Can you work these out from the model? Positions are in its coordinate system, mm. A direction names the side the tool comes from. Give positions to 0.01 mm unless a question says otherwise; leave off trailing zeros. Order: outer loops, then holes, each group sorted by start corner. A loop starts at its lowest first (then second) coordinate and runs counter-clockwise, first axis right, second up. Notation, with made-up numbers: M 66,51 L 121,51 A28 ccw 121,77 Z; hole C -11,-13 d8. An arc over 180 degrees is marked long. Use one line per item in the form item = value. Start each with the question number.
1. I want a section at B-B, the plane z = -39.5. List the corners of the cut face in (x, y) for me, and give its area (3 significant figures).
2. For faces 1 (the face through (48.57, 26.55, -25.74)), 2 (the face through (25, 29, -2)), 3 (the face through (37, 29, -30)), which set-ups out of +Z, -Z, +X, -X, +Y, -Y let a thin tool reach every point of the face, with its end or its side?
3. I want a section at A-A, the plane y = 11. List the corners of the cut face in (x, z) for me.
4. Will these pins go through, and if not, where does the flat tip stop? P1, Ø0.6, axis at x = 22.5, z = -49.5, coming from the +Y side; P2, Ø5, axis at x = 22.98, z = -29.85, coming from the -Y side; P3, Ø5, axis at x = 43.5, z = -40.5, coming from the +Y side; P4, Ø7.5, axis at x = 19.5, y = 12, coming from the -Z side.
5. We'd pull the mould along Y, two halves only. Please class faces 4 (the face through (22, 12, -50.2)), 5 (the face through (21.53, 29.51, -31.22)), 6 (the face through (25.74, 26.55, -2.43)): +Y half, -Y half, draft (parallel to the pull), parting line (faces both ways), or undercut.
6. I need wall thicknesses on L1, parallel to Z at x = 18, y = 22; L2, parallel to Z at x = 26, y = 4; L3, parallel to X at y = 16, z = -24. Which ranges of each line are inside material? Lowest first, please.
7. I want a section at C-C, the plane x = 44.25. Count the separate pieces of the cut face and the enclosed holes in it, and give its area (3 significant figures).
```python
from build123d import *

# Parameters (mm, degrees)
BOSS_EXTRUDE1_DEPTH = 30
CUT_EXTRUDE1_DEPTH  = 27
SKETCH3_R           = 1.75
SKETCH3_R_2         = 1.25
CUT_EXTRUDE2_DEPTH  = 3
SKETCH4_R           = 3
SKETCH4_R_2         = 2
CUT_EXTRUDE3_DEPTH  = 1
CUT_EXTRUDE4_DEPTH  = 2
FILLET1_R           = 5
FILLET2_R           = 1.5
SKETCH6_R           = 1
CUT_EXTRUDE5_DEPTH  = 1
CUT_EXTRUDE6_DEPTH  = 0.8


with BuildPart() as part:
    # Sketch1 → Boss-Extrude1 (new body)
    with BuildSketch(Plane(origin=(0, 0, 0), x_dir=(1, 0, 0), z_dir=(0, 1, 0))):
        with BuildLine():
            Line((8, 0), (43, 0))
            ThreePointArc((43, 0), (48.656854249, 2.343145751), (51, 8))
            Line((51, 8), (51, 43))
            ThreePointArc((51, 43), (48.656854249, 48.656854249), (43, 51))
            Line((43, 51), (8, 51))
            ThreePointArc((8, 51), (2.343145751, 48.656854249), (0, 43))
            Line((0, 43), (0, 8))
            ThreePointArc((0, 8), (2.343145751, 2.343145751), (8, 0))
        make_face()
    extrude(amount=BOSS_EXTRUDE1_DEPTH)

    # Sketch2 → Cut-Extrude1 (cut)
    with BuildSketch(Plane.XZ):
        with BuildLine():
            Line((8, -2), (43, -2))
            ThreePointArc((43, -2), (47.242640687, -3.757359313), (49, -8))
            Line((49, -8), (49, -43))
            ThreePointArc((49, -43), (47.242640687, -47.242640687), (43, -49))
            Line((43, -49), (8, -49))
            ThreePointArc((8, -49), (3.757359313, -47.242640687), (2, -43))
            Line((2, -43), (2, -8))
            ThreePointArc((2, -8), (3.757359313, -3.757359313), (8, -2))
        make_face()
    extrude(amount=-CUT_EXTRUDE1_DEPTH, mode=Mode.SUBTRACT)

    # Sketch3 → Cut-Extrude2 (cut)
    with BuildSketch(Plane.XZ.offset(-27)):
        with Locations(Location((6.75, -11.5, 0), (0, 0, 270))):
            Circle(SKETCH3_R)
        with Locations(Location((44.25, -11.5, 0), (0, 0, 90))):
            Circle(SKETCH3_R)
        with Locations(Location((44.25, -39.5, 0), (0, 0, 270))):
            Circle(SKETCH3_R)
        with Locations(Location((6.75, -39.5, 0), (0, 0, 90))):
            Circle(SKETCH3_R)
        with Locations(Location((38.655, -12.5, 0), (0, 0, 270))):
            Circle(SKETCH3_R_2)
        with Locations(Location((12.585, -12.5, 0), (0, 0, 270))):
            Circle(SKETCH3_R_2)
    extrude(amount=-CUT_EXTRUDE2_DEPTH, mode=Mode.SUBTRACT)

    # Sketch4 → Cut-Extrude3 (cut)
    with BuildSketch(Plane(origin=(0, 30, 0), x_dir=(1, 0, 0), z_dir=(0, 1, 0))):
        with Locations(Location((44.25, 39.5, 0), (0, 0, 270))):
            Circle(SKETCH4_R)
        with Locations(Location((6.75, 39.5, 0), (0, 0, 270))):
            Circle(SKETCH4_R)
        with Locations(Location((6.75, 11.5, 0), (0, 0, 270))):
            Circle(SKETCH4_R)
        with Locations(Location((12.585, 12.5, 0), (0, 0, 270))):
            Circle(SKETCH4_R_2)
        with Locations(Location((38.655, 12.5, 0), (0, 0, 270))):
            Circle(SKETCH4_R_2)
        with Locations(Location((44.25, 11.5, 0), (0, 0, 270))):
            Circle(SKETCH4_R)
    extrude(amount=-CUT_EXTRUDE3_DEPTH, mode=Mode.SUBTRACT)

    # Sketch5 → Cut-Extrude4 (cut)
    with BuildSketch(Plane.XY.offset(-49)):
        with BuildLine():
            Line((9.585, 18), (34.085, 18))
            ThreePointArc((34.085, 18), (34.792106781, 17.707106781), (35.085, 17))
            Line((35.085, 17), (35.085, 14))
            ThreePointArc((35.085, 14), (34.792106781, 13.292893219), (34.085, 13))
            Line((34.085, 13), (9.585, 13))
            ThreePointArc((9.585, 13), (8.877893219, 13.292893219), (8.585, 14))
            Line((8.585, 14), (8.585, 17))
            ThreePointArc((8.585, 17), (8.877893219, 17.707106781), (9.585, 18))
        make_face()
    extrude(amount=-CUT_EXTRUDE4_DEPTH, mode=Mode.SUBTRACT)

    # Fillet1
    # the kernel refuses this fillet: 5 mm, written as the material it takes off along each edge
    with BuildSketch(Plane(origin=(8, 30, -43), x_dir=(0, 0, -1), z_dir=(1, 0, 0))) as fillet1_piece_1:
        with BuildLine():
            CenterArc((8 - FILLET1_R, -FILLET1_R), FILLET1_R, 0, 90)
            Line((8 - FILLET1_R, 0), (8, 0))
            Line((8, 0), (8, -FILLET1_R))
        make_face()
    revolve(axis=Axis((8, 30, -43), (0, 1, 0)), revolution_arc=90, mode=Mode.SUBTRACT)
    with BuildSketch(Plane(origin=(0, 30, -43), x_dir=(0, -1, 0), z_dir=(0, 0, 1))) as fillet1_piece_2:
        with BuildLine():
            CenterArc((FILLET1_R, FILLET1_R), FILLET1_R, 180, 90)
            Line((0, FILLET1_R), (0, 0))
            Line((0, 0), (FILLET1_R, 0))
        make_face()
    extrude(amount=35, mode=Mode.SUBTRACT)
    with BuildSketch(Plane(origin=(8, 30, -8), x_dir=(-1, 0, 0), z_dir=(0, 0, -1))) as fillet1_piece_3:
        with BuildLine():
            CenterArc((8 - FILLET1_R, -FILLET1_R), FILLET1_R, 0, 90)
            Line((8 - FILLET1_R, 0), (8, 0))
            Line((8, 0), (8, -FILLET1_R))
        make_face()
    revolve(axis=Axis((8, 30, -8), (0, 1, 0)), revolution_arc=90, mode=Mode.SUBTRACT)
    with BuildSketch(Plane(origin=(8, 30, 0), x_dir=(0, 0, -1), z_dir=(1, 0, 0)), Plane(origin=(51, 30, -8), x_dir=(-1, 0, 0), z_dir=(0, 0, -1)), Plane(origin=(43, 30, -51), x_dir=(0, 0, 1), z_dir=(-1, 0, 0))) as fillet1_piece_4:
        with BuildLine():
            CenterArc((FILLET1_R, -FILLET1_R), FILLET1_R, 90, 90)
            Line((0, -FILLET1_R), (0, 0))
            Line((0, 0), (FILLET1_R, 0))
        make_face()
    extrude(amount=35, mode=Mode.SUBTRACT)
    with BuildSketch(Plane(origin=(43, 30, -8), x_dir=(0, 0, 1), z_dir=(-1, 0, 0))) as fillet1_piece_5:
        with BuildLine():
            CenterArc((8 - FILLET1_R, -FILLET1_R), FILLET1_R, 0, 90)
            Line((8, -FILLET1_R), (8, 0))
            Line((8, 0), (8 - FILLET1_R, 0))
        make_face()
    revolve(axis=Axis((43, 30, -8), (0, 1, 0)), revolution_arc=90, mode=Mode.SUBTRACT)
    with BuildSketch(Plane(origin=(43, 30, -43), x_dir=(1, 0, 0), z_dir=(0, 0, 1))) as fillet1_piece_6:
        with BuildLine():
            CenterArc((8 - FILLET1_R, -FILLET1_R), FILLET1_R, 0, 90)
            Line((8, -FILLET1_R), (8, 0))
            Line((8, 0), (8 - FILLET1_R, 0))
        make_face()
    revolve(axis=Axis((43, 30, -43), (0, 1, 0)), revolution_arc=90, mode=Mode.SUBTRACT)

    # Fillet2
    fillet2_edges = [part.edges().sort_by_distance(p)[0] for p in [
        (47.242640687, 27, -47.242640687),
        (25.5, 27, -49),
        (3.757359313, 27, -47.242640687),
        (2, 27, -25.5),
        (3.757359313, 27, -3.757359313),
        (25.5, 27, -2),
        (47.242640687, 27, -3.757359313),
        (49, 27, -25.5),
    ]]
    fillet(fillet2_edges, radius=FILLET2_R)

    # Sketch6 → Cut-Extrude5 (cut)
    # profile 1 of 4: a face of its own
    with BuildSketch(Plane(origin=(0, 30, 0), x_dir=(1, 0, 0), z_dir=(0, 1, 0))):
        with BuildLine():
            Line((24.920410097, 30.348440054), (31.776811643, 30.348440054))
            Line((31.776811643, 30.348440054), (30.50904469, 31.616207007))
            ThreePointArc((30.50904469, 31.616207007), (30.50904469, 32.323313788), (31.216151471, 32.323313788))
            Line((31.216151471, 32.323313788), (33.337471815, 30.201993444))
            ThreePointArc((33.337471815, 30.201993444), (33.483918424, 29.848440054), (33.337471815, 29.494886663))
            Line((33.337471815, 29.494886663), (31.216151471, 27.37356632))
            ThreePointArc((31.216151471, 27.37356632), (30.50904469, 27.37356632), (30.50904469, 28.080673101))
            Line((30.50904469, 28.080673101), (31.776811643, 29.348440054))
            Line((31.776811643, 29.348440054), (24.920410097, 29.348440054))
            ThreePointArc((24.920410097, 29.348440054), (24.398131986, 28.434226491), (23.483918424, 27.911948381))
            Line((23.483918424, 27.911948381), (23.483918424, 21.055546835))
            Line((23.483918424, 21.055546835), (24.751685377, 22.323313788))
            ThreePointArc((24.751685377, 22.323313788), (25.458792158, 22.323313788), (25.458792158, 21.616207007))
            Line((25.458792158, 21.616207007), (23.337471815, 19.494886663))
            ThreePointArc((23.337471815, 19.494886663), (22.983918424, 19.348440054), (22.630365033, 19.494886663))
            Line((22.630365033, 19.494886663), (20.50904469, 21.616207007))
            ThreePointArc((20.50904469, 21.616207007), (20.50904469, 22.323313788), (21.216151471, 22.323313788))
            Line((21.216151471, 22.323313788), (22.483918424, 21.055546835))
            Line((22.483918424, 21.055546835), (22.483918424, 27.911948381))
            ThreePointArc((22.483918424, 27.911948381), (21.569704862, 31.262653616), (24.920410097, 30.348440054))
        make_face()
        with Locations(Location((22.983918424, 29.848440054, 0), (0, 0, 270))):
            Circle(SKETCH6_R, mode=Mode.SUBTRACT)
    # profile 2 of 4: a face of its own
    with BuildSketch(Plane(origin=(0, 30, 0), x_dir=(1, 0, 0), z_dir=(0, 1, 0))):
        with BuildLine():
            Line((20.166103424, 34.766202804), (15.455317355, 34.766202804))
            ThreePointArc((15.455317355, 34.766202804), (14.955317355, 34.266202804), (15.455317355, 33.766202804))
            Line((15.455317355, 33.766202804), (17.751889862, 33.766202804))
            Line((17.751889862, 33.766202804), (14.569909347, 30.584222289))
            Line((14.569909347, 30.584222289), (19.277016128, 30.584222289))
            ThreePointArc((19.277016128, 30.584222289), (19.777016128, 31.084222289), (19.277016128, 31.584222289))
            Line((19.277016128, 31.584222289), (16.984122909, 31.584222289))
            Line((16.984122909, 31.584222289), (20.166103424, 34.766202804))
        make_face()
    # profile 3 of 4: a face of its own
    with BuildSketch(Plane(origin=(0, 30, 0), x_dir=(1, 0, 0), z_dir=(0, 1, 0))):
        with BuildLine():
            Line((37.725215013, 30.056361033), (37.725215013, 32.349254251))
            ThreePointArc((37.725215013, 32.349254251), (37.225215013, 32.849254251), (36.725215013, 32.349254251))
            Line((36.725215013, 32.349254251), (36.725215013, 30.056361033))
            Line((36.725215013, 30.056361033), (35.103894669, 28.435040689))
            ThreePointArc((35.103894669, 28.435040689), (35.103894669, 27.727933908), (35.81100145, 27.727933908))
            Line((35.81100145, 27.727933908), (37.225215013, 29.14214747))
            Line((37.225215013, 29.14214747), (38.639428575, 27.727933908))
            ThreePointArc((38.639428575, 27.727933908), (39.346535356, 27.727933908), (39.346535356, 28.435040689))
            Line((39.346535356, 28.435040689), (37.725215013, 30.056361033))
        make_face()
    # profile 4 of 4: a face of its own
    with BuildSketch(Plane(origin=(0, 30, 0), x_dir=(1, 0, 0), z_dir=(0, 1, 0))):
        with BuildLine():
            Line((23.864017642, 16.318192841), (25.278231204, 17.732406403))
            ThreePointArc((25.278231204, 17.732406403), (25.278231204, 18.439513185), (24.571124423, 18.439513185))
            Line((24.571124423, 18.439513185), (23.15691086, 17.025299622))
            Line((23.15691086, 17.025299622), (21.742697298, 18.439513185))
            ThreePointArc((21.742697298, 18.439513185), (21.035590517, 18.439513185), (21.035590517, 17.732406403))
            Line((21.035590517, 17.732406403), (22.449804079, 16.318192841))
            Line((22.449804079, 16.318192841), (21.035590517, 14.903979279))
            ThreePointArc((21.035590517, 14.903979279), (21.035590517, 14.196872497), (21.742697298, 14.196872497))
            Line((21.742697298, 14.196872497), (23.15691086, 15.61108606))
            Line((23.15691086, 15.61108606), (24.571124423, 14.196872497))
            ThreePointArc((24.571124423, 14.196872497), (25.278231204, 14.196872497), (25.278231204, 14.903979279))
            Line((25.278231204, 14.903979279), (23.864017642, 16.318192841))
        make_face()
    extrude(amount=-CUT_EXTRUDE5_DEPTH, mode=Mode.SUBTRACT)

    # Sketch7 → Cut-Extrude6 (cut)
    with BuildSketch(Plane(origin=(0, 0, -51), x_dir=(-1, 0, 0), z_dir=(0, 0, -1))):
        with BuildLine():
            Line((-35.085, 23), (-8.585, 23))
            ThreePointArc((-8.585, 23), (-5.049466094, 21.535533906), (-3.585, 18))
            Line((-3.585, 18), (-3.585, 13))
            ThreePointArc((-3.585, 13), (-5.049466094, 9.464466094), (-8.585, 8))
            Line((-8.585, 8), (-35.085, 8))
            ThreePointArc((-35.085, 8), (-38.620533906, 9.464466094), (-40.085, 13))
            Line((-40.085, 13), (-40.085, 18))
            ThreePointArc((-40.085, 18), (-38.620533906, 21.535533906), (-35.085, 23))
        make_face()
    extrude(amount=-CUT_EXTRUDE6_DEPTH, mode=Mode.SUBTRACT)


solid = part.part
```
Check result:
q1.outline = M 0,0 L 2,0 L 2,25.5 A1.5 cw 3.5,27 L 5,27 L 5,29 L 3.75,29 L 3.75,29.84 A5 ccw 0,25 Z; M 8.5,27 L 42.5,27 L 42.5,29 L 41.25,29 L 41.25,30 L 9.75,30 L 9.75,29 L 8.5,29 Z; M 46,27 L 47.5,27 A1.5 cw 49,25.5 L 49,0 L 51,0 L 51,25 A5 ccw 47.25,29.84 L 47.25,29 L 46,29 Z
q1.area = 225 mm2
q2.face_1 = -Y
q2.face_2 = +Z, +X, -X, +Y
q2.face_3 = +Y
q3.outline = M 0,-43 A8 ccw 4.51,-50.2 L 39.67,-50.2 L 39.67,-51 L 43,-51 A8 ccw 51,-43 L 51,-8 A8 ccw 43,0 L 8,0 A8 ccw 0,-8 Z; hole M 2,-43 A6 ccw 8,-49 L 43,-49 A6 ccw 49,-43 L 49,-8 A6 ccw 43,-2 L 8,-2 A6 ccw 2,-8 Z
q4.P1 = 28.84
q4.P2 = 27
q4.P3 = 30
q4.P4 = -50.2
q5.face_4 = undercut
q5.face_5 = draft
q5.face_6 = -Y half
q6.L1 = -50.2 to -49, -2 to 0
q6.L2 = -51 to -49, -2 to 0
q6.L3 = 0 to 2, 49 to 51
q7.separate_pieces = 3
q7.enclosed_holes = 0
q7.area = 226 mm2
